```python
from build123d import *

# Parameters (mm, degrees)
SKETCH1_W           = 50
SKETCH1_H           = 22
BOSS_EXTRUDE1_DEPTH = 22.6
SKETCH3_R           = 5
BOSS_EXTRUDE2_DEPTH = 12.5


with BuildPart() as part:
    # Sketch1 → Boss-Extrude1 (new body)
    with BuildSketch(Plane.XY):
        Rectangle(SKETCH1_W, SKETCH1_H)
    extrude(amount=BOSS_EXTRUDE1_DEPTH)

    # Sketch3 → Boss-Extrude2 (add, symmetric)
    with BuildSketch(Plane(origin=(0, 0, 0), x_dir=(0, 0, -1), z_dir=(1, 0, 0))):
        with BuildLine():
            Line((-22.6, 11), (-22.6, 21))
            ThreePointArc((-22.6, 21), (-11.3, 32.3), (0, 21))
            Line((0, 21), (0, 11))
            Line((0, 11), (-22.6, 11))
        make_face()
        with Locations((-11.3, 24)):
            Circle(SKETCH3_R, mode=Mode.SUBTRACT)
    boss_extrude2 = extrude(amount=BOSS_EXTRUDE2_DEPTH, both=True)

    # Mirror1: Boss-Extrude2 across plane
    add(boss_extrude2.mirror(Plane.ZX))


solid = part.part
```
Geometry check sheet. Reference: the model listing, model coordinates, mm. A direction names the side the tool comes from. Give positions to 0.01 mm unless a question says otherwise; leave off trailing zeros. Loops run counter-clockwise (first coordinate to the right, second up) from the corner with the lowest first, then second, coordinate; pieces in that order, holes last. Notation, with made-up numbers: M -18,-15 L 14,-15 A20 ccw 14,19 Z; hole C -0.5,-21.5 d3. An arc over 180 degrees is marked long. Write item = value, one per line. Start each with the question number.
1. Section check A-A, the plane z = 11.3. Enter the section's corners in (x, y), plus the area to 4 significant figures.
2. Tool access check on faces 1 (the face through (-19, -11, 11)), 2 (the face through (-12.5, 19, 9)), 3 (the face through (12.5, 19, 9)), 4 (the face through (0.2, 32.3, 11.5)), 5 (the face through (12.5, -19, 9)). Record the directions out of +Z, -Z, +X, -X, +Y, -Y that give a thin tool (end or side, any length) a straight path to the whole face; none if there is none.
3. Section check C-C, the plane x = -8. Enter the section's corners in (y, z).
4. Section check B-B, the plane y = 24. Enter the section's corners in (x, z), plus the area to 3 significant figures.
5. Section check D-D, the plane x = 20.5. Enter the section's corners in (y, z).
6. Go/stop test with flat-tipped pins: P1, Ø8, axis at y = -24, z = 16, coming from the -X side; P2, Ø4, axis at x = -19, z = 16.5, coming from the -Y side; P3, Ø12, axis at x = -8.5, z = 10.5, coming from the -Y side; P4, Ø6.5, axis at y = 26, z = 7.5, coming from the +X side. Record where each tip stops, or that it passes through.
7. Thickness scan on probe 1 along Y at (x, z) = (-1.75, 11.3); probe 2 along Y at (x, z) = (-21.5, 5); probe 3 along Z at (x, y) = (-2.5, -24). Record the ranges inside material, lowest first.
8. Draft check along Z on faces 6 (the face through (0, 0, 22.6)), 7 (the face through (-0.18, 19.12, 12.38)), 8 (the face through (-25, 0, 11)). Enter one of: +Z half, -Z half, draft (parallel to the pull), parting line (faces both ways), or undercut.
Values follow:
q1.outline = M -25,-11 L -12.5,-11 L -12.5,-19 L 12.5,-19 L 12.5,-11 L 25,-11 L 25,11 L 12.5,11 L 12.5,19 L -12.5,19 L -12.5,11 L -25,11 Z; M -12.5,-32.3 L 12.5,-32.3 L 12.5,-29 L -12.5,-29 Z; M -12.5,29 L 12.5,29 L 12.5,32.3 L -12.5,32.3 Z
q1.area = 1,665 mm^2
q2.face_1 = +Z, -Z, -X, -Y
q2.face_2 = +Z, -Z, -X, +Y
q2.face_3 = +Z, -Z, +X, +Y
q2.face_4 = +X, -X, +Y
q2.face_5 = +Z, -Z, +X, -Y
q3.outline = M -21,0 L 21,0 A11.3 ccw 21,22.6 L -21,22.6 A11.3 ccw Z; hole C -24,11.3 d10; hole C 24,11.3 d10
q4.outline = M -12.5,0.41 L 12.5,0.41 L 12.5,6.3 L -12.5,6.3 Z; M -12.5,16.3 L 12.5,16.3 L 12.5,22.19 L -12.5,22.19 Z
q4.area = 295 mm^2
q5.outline = M -11,0 L 11,0 L 11,22.6 L -11,22.6 Z
q6.P1 = -12.5
q6.P2 = -11
q6.P3 = -32.3
q6.P4 = 12.5
q7.probe_1 = -32.3 to -29, -19 to 19, 29 to 32.3
q7.probe_2 = -11 to 11
q7.probe_3 = 0.41 to 6.3, 16.3 to 22.19
q8.face_6 = +Z half
q8.face_7 = undercut
q8.face_8 = draft
